Can you work these out from the drawing? Everything is in mm from the part's minimum corner. Give positions to 0.01 mm unless a question says otherwise; leave off trailing zeros. Order: outer loops, then holes, each group sorted by start corner. A loop starts at its lowest first (then second) coordinate and runs counter-clockwise, first axis right, second up. Notation, with made-up numbers: (13, 83.25) -> (69, 83.25) arc R16 cw to (69, 99.25) -> close; hole circle Ø6 at (-7.5, 71.25). An arc over 180 degrees is marked (long way). Answer as CSV lines item,"result". Start each with the question number.
(1) I want a section at B-B (x = 8.75). Please give me the cut outline in (y, z), plus the area to 3 significant figures.
(2) I want a section at C-C (z = 26.25). Please give me the cut outline in (x, y), plus the area to 3 significant figures.
(3) I want a section at A-A (y = 13.5). Please give me the cut outline in (x, z), plus the area to 3 significant figures.
(4) Will this pin go through, and if not, where does the flat tip stop? pin 1 Ø6 at (y, z) = (4, 25.5) entering from -X.
(5) I need wall thicknesses on L1, parallel to Z at x = 12.25, y = 15; L2, parallel to Z at x = 6.5, y = 2.25; L3, parallel to X at y = 15.25, z = 22.75. Which ranges of each line are inside material? Lowest first, please.
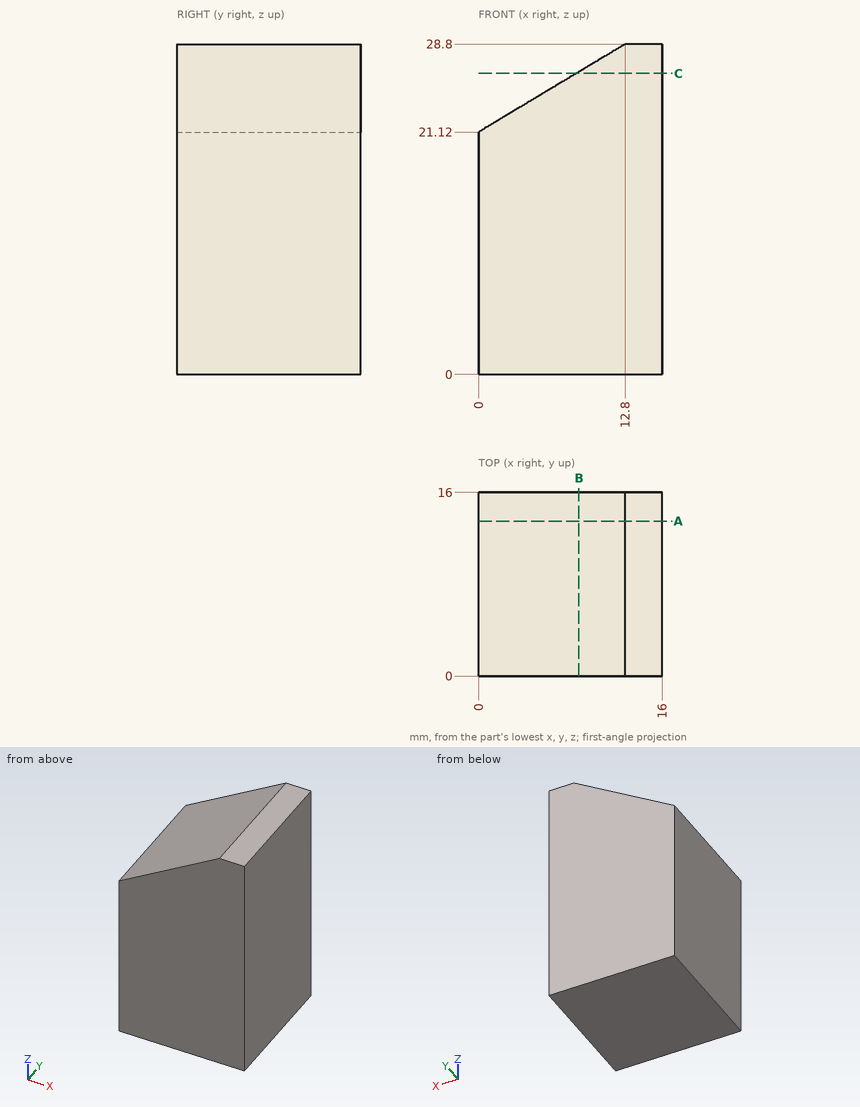
Final values:
1,outline,"(0, 0) -> (16, 0) -> (16, 26.37) -> (0, 26.37) -> close"
1,area,"422 mm²"
2,outline,"(8.55, 0) -> (16, 0) -> (16, 16) -> (8.55, 16) -> close"
2,area,"119 mm²"
3,outline,"(0, 0) -> (16, 0) -> (16, 28.8) -> (12.8, 28.8) -> (0, 21.12) -> close"
3,area,"412 mm²"
4,pin 1,"x = 2.3"
5,L1,"0 to 28.47"
5,L2,"0 to 25.02"
5,L3,"2.72 to 16"
